Geometry: final body of the model. Coordinates: model frame, mm. Face numbers are marked on the shaded views. A direction names the side the tool comes from. Round coordinates to 2 decimals unless told otherwise and drop trailing zeros. Order: outer loops, then holes, each group sorted by start corner. A loop starts at its lowest first (then second) coordinate and runs counter-clockwise, first axis right, second up. Notation, with made-up numbers: M -28.5,-37.5 L -14.5,-37.5 A25 ccw -14.5,-3.5 Z; hole C 73,11 d3. An arc over 180 degrees is marked long. Put each result on its own line as item: value. Start each with the question number.
1) First-contact query: P1, Ø12, axis at x = 16, y = 50, coming from the -Z side; P2, Ø3.5, axis at x = 86, y = 20, coming from the +Z side; P3, Ø3, axis at x = 72, y = 44.5, coming from the +Z side. Flat tips, straight axial feed; report the tip coordinate or a pass-through.
2) Draft query along X for the marked faces 1, 2 and 3. Return one class per face: pulls with the +X half, pulls with the -X half, needs draft (parallel to the pull), parting line crosses it, or undercut.
3) Material intervals for probe 1 along X at (y, z) = (49, 9.75); probe 2 along Y at (x, z) = (75, 5); probe 3 along Y at (x, z) = (8, 4), sorted ascending. Write a range as [from, to].
4) Section A-A, the plane z = 4.75. Return loops of the section in (x, y), then the cut area to 3 significant figures.
5) Access query for the marked faces 4 and 5. Directions: +Z, -Z, +X, -X, +Y, -Y. A direction counts if a zero-diameter tool reaches every point of the face in a straight line with its end or side. Return the directions, or none.
6) Section D-D, the plane x = 6. Return loops of the section in (y, z), then the cut area to 3 significant figures.
7) Section C-C, the plane x = 44.5. Return loops of the section in (y, z), then the cut area to 3 significant figures.
8) Section B-B, the plane y = 15. Return loops of the section in (x, z), then the cut area to 3 significant figures.
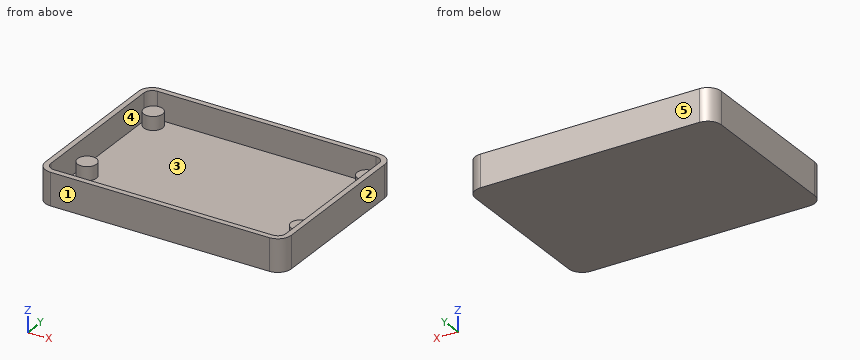
from build123d import *

# Parameters (mm, degrees)
PAD_DEPTH                    = 12
POCKET_DEPTH                 = 10
SKETCH003_R                  = 3.5
PAD001_DEPTH                 = 5
SKETCH003_LINEARPATTERN_2_R  = 3.5
PAD001_LINEARPATTERN_2_DEPTH = 5
LINEARPATTERN001_COUNT       = 2
LINEARPATTERN001_PITCH       = 39


with BuildPart() as part:
    # Sketch → Pad (new body)
    with BuildSketch(Plane.XY):
        with BuildLine():
            Line((5, 0), (86, 0))
            ThreePointArc((86, 0), (89.535534, 1.464466), (91, 5))
            Line((91, 5), (91, 60))
            ThreePointArc((91, 60), (89.535534, 63.535534), (86, 65))
            Line((86, 65), (5, 65))
            ThreePointArc((5, 65), (1.464466, 63.535534), (0, 60))
            Line((0, 60), (0, 5))
            ThreePointArc((0, 5), (1.464466, 1.464466), (5, 0))
        make_face()
    extrude(amount=PAD_DEPTH)

    # Sketch002 → Pocket (cut)
    with BuildSketch(Plane.XY.offset(12)):
        with BuildLine():
            Line((5, 2), (86, 2))
            ThreePointArc((86, 2), (88.12132, 2.87868), (89, 5))
            Line((89, 5), (89, 60))
            ThreePointArc((89, 60), (88.12132, 62.12132), (86, 63))
            Line((86, 63), (5, 63))
            ThreePointArc((5, 63), (2.87868, 62.12132), (2, 60))
            Line((2, 60), (2, 5))
            ThreePointArc((2, 5), (2.87868, 2.87868), (5, 2))
        make_face()
    extrude(amount=-POCKET_DEPTH, mode=Mode.SUBTRACT)

    # Sketch003 → Pad001 (join)
    with BuildSketch(Plane.XY.offset(2)):
        with Locations((6, 20)):
            Circle(SKETCH003_R)
    pad001 = extrude(amount=PAD001_DEPTH)

    # Sketch003 LinearPattern 2 → Pad001 LinearPattern 2 (add)
    with BuildSketch(Plane(origin=(79, 0, 2), x_dir=(1, 0, 0), z_dir=(0, 0, 1))):
        with Locations((6, 20)):
            Circle(SKETCH003_LINEARPATTERN_2_R)
    pad001_linearpattern_2 = extrude(amount=PAD001_LINEARPATTERN_2_DEPTH)

    # LinearPattern001: Pad001, Pad001 LinearPattern 2 ×2
    with Locations(*[(0, i * LINEARPATTERN001_PITCH, 0) for i in range(1, LINEARPATTERN001_COUNT)]):
        add(pad001)
        add(pad001_linearpattern_2)


solid = part.part
Result sheet:
1. P1: stops at z = 0
1. P2: stops at z = 7
1. P3: stops at z = 2
2. face 1: needs draft
2. face 2: pulls with the +X half
2. face 3: undercut
3. probe 1: x = [0, 2], [89, 91]
3. probe 2: y = [0, 2], [63, 65]
3. probe 3: y = [0, 2], [17.13, 22.87], [56.13, 61.87], [63, 65]
4. outline: M 0,5 A5 ccw 5,0 L 86,0 A5 ccw 91,5 L 91,60 A5 ccw 86,65 L 5,65 A5 ccw 0,60 Z; C 6,20 d7; C 6,59 d7; C 85,20 d7; C 85,59 d7; hole M 2,5 A3 ccw 5,2 L 86,2 A3 ccw 89,5 L 89,60 A3 ccw 86,63 L 5,63 A3 ccw 2,60 Z
4. area: 748 mm2
5. face 4: +Z
5. face 5: +Z, -Z, +X, -X, +Y
6. outline: M 0,0 L 65,0 L 65,12 L 63,12 L 63,2 L 62.5,2 L 62.5,7 L 55.5,7 L 55.5,2 L 23.5,2 L 23.5,7 L 16.5,7 L 16.5,2 L 2,2 L 2,12 L 0,12 Z
6. area: 240 mm2
7. outline: M 0,0 L 65,0 L 65,12 L 63,12 L 63,2 L 2,2 L 2,12 L 0,12 Z
7. area: 170 mm2
8. outline: M 0,0 L 91,0 L 91,12 L 89,12 L 89,2 L 2,2 L 2,12 L 0,12 Z
8. area: 222 mm2
